The listing builds one solid part. Answer for the finished solid, in the listing's coordinates (mm). Face numbers are marked on the shaded views. A direction names the side the tool comes from. Give positions to 0.01 mm unless a question says otherwise; leave off trailing zeros. Write each loop counter-clockwise with the first axis right and the second up, starting at its lowest first coordinate (ties: lowest second). Pieces come first, ordered by that corner, then holes. Notation, with made-up numbers: (85.5, 75) - (99.5, 75) arc R20 ccw to (99.5, 91) - close; hole circle Ø4 at (56, 1.5). An arc over 180 degrees is marked (long way). Answer as CSV lines item,"result". Start each with the question number.
(1) Each of these flat-tipped pins is pushed along its axis until it touches: pin 1 Ø0.8 at (y, z) = (1, 1.5) entering from +X; pin 2 Ø1.5 at (x, y) = (-5, -3.5) entering from -Z; pin 3 Ø1.4 at (y, z) = (1.5, -1) entering from -X. Where does it stop, or does it pass through?
(2) Find section D-D (x = 1.5). Write down the section's boundary in (y, z), then the cut area to 3 significant figures.
(3) Find section A-A (y = 1.5). Write down the section's boundary in (x, z), then the cut area to 3 significant figures.
(4) Straight lines are drawn through the part: probe 1 along Z at (x, y) = (0, -3.75); probe 2 along Y at (x, z) = (5.25, -0.35); probe 3 along Z at (x, y) = (2.75, -2.5). For each, find the intervals that lie inside material, in ascending order.
(5) Find section C-C (z = -1.15). Write down the section's boundary in (x, y).
(6) For the marked faces 1, 2 and 3, determine the directions among +Z, -Z, +X, -X, +Y, -Y from which every point of the face is accessible in a straight line to the end or side of a thin tool.
(7) Find section B-B (x = 4.75). Write down the section's boundary in (y, z).
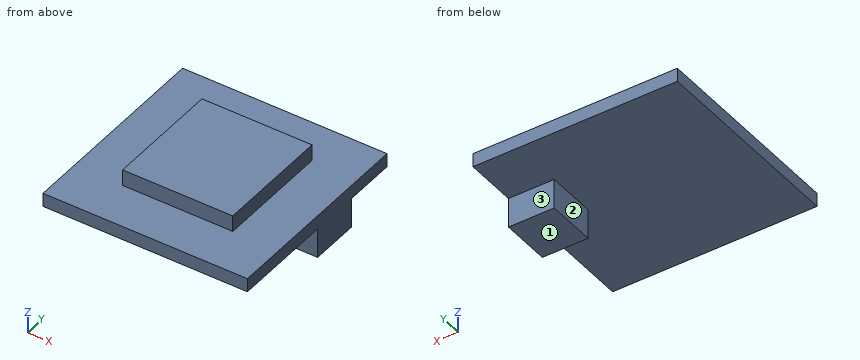
from build123d import *

# Parameters (mm, degrees)
F0_W     = 6.464736
F0_H     = 6.81608
F0_W_2   = 2.685256
F0_H_2   = 2.91172
F1_DEPTH = 0.8
F2_DEPTH = 1.75
F3_DEPTH = 1.75


with BuildPart() as f1:
    # F0 (on Top) → F1 (new body)
    with BuildSketch(Plane.XY):
        Polygon((5.88367, 5.962724), (-6.11633, 5.962724), (-6.11633, -6.037276), (5.88367, -6.037276), (5.88367, 0), (3.198414, 0), (3.198414, 2.91172), (5.88367, 2.91172), align=None)
        with Locations((-0.049542, 0.065831)):
            Rectangle(F0_W, F0_H, mode=Mode.SUBTRACT)
        with Locations((4.541042, 1.45586)):
            Rectangle(F0_W_2, F0_H_2)
        with Locations((-0.049542, 0.065831)):
            Rectangle(F0_W, F0_H)
    extrude(amount=F1_DEPTH)

    # F0 (on Top) → F2 (join)
    with BuildSketch(Plane.XY):
        with Locations((-0.049542, 0.065831)):
            Rectangle(F0_W, F0_H)
    extrude(amount=F2_DEPTH)

    # F0 (on Top) → F3 (join)
    with BuildSketch(Plane.XY):
        with Locations((4.541042, 1.45586)):
            Rectangle(F0_W_2, F0_H_2)
    extrude(amount=-F3_DEPTH)


solid = f1.part
Result set:
1,pin 1,"x = 3.18"
1,pin 2,"z = 0"
1,pin 3,"x = 3.2"
2,outline,"(-6.04, 0) - (5.96, 0) - (5.96, 0.8) - (3.47, 0.8) - (3.47, 1.75) - (-3.34, 1.75) - (-3.34, 0.8) - (-6.04, 0.8) - close"
2,area,"16.1 mm^2"
3,outline,"(-6.12, 0) - (3.2, 0) - (3.2, -1.75) - (5.88, -1.75) - (5.88, 0.8) - (3.18, 0.8) - (3.18, 1.75) - (-3.28, 1.75) - (-3.28, 0.8) - (-6.12, 0.8) - close"
3,area,"20.4 mm^2"
4,probe 1,"0 to 0.8"
4,probe 2,"0 to 2.91"
4,probe 3,"0 to 1.75"
5,outline,"(3.2, 0) - (5.88, 0) - (5.88, 2.91) - (3.2, 2.91) - close"
6,face 1,"-Z, +X, -X, +Y, -Y"
6,face 2,"-Z, -X, +Y, -Y"
6,face 3,"-Z, +X, -X, +Y"
7,outline,"(-6.04, 0) - (0, 0) - (0, -1.75) - (2.91, -1.75) - (2.91, 0) - (5.96, 0) - (5.96, 0.8) - (-6.04, 0.8) - close"
